Design review of the part built by this model. Coordinates are the model's own, in mm. Face numbers are marked on the shaded views. A direction names the side the tool comes from. Give positions to 0.01 mm unless a question says otherwise; leave off trailing zeros. Loops run counter-clockwise (first coordinate to the right, second up) from the corner with the lowest first, then second, coordinate; pieces in that order, holes last. Notation, with made-up numbers: (19.5, 24.25) -> (62.5, 24.25) arc R24 cw to (62.5, 56.25) -> close; hole circle Ø10 at (6, -9). An arc over 180 degrees is marked (long way). Use a Markdown table: item, result. Add a question column.
1. To check wall thickness, follow line 1 (Y direction, x = 0, z = 11); line 2 (Y direction, x = 0, z = 0.7). State the ranges of each line that lie inside material, in increasing order.
2. For pin 1 Ø3 at (y, z) = (24, 6.5) entering from -X; pin 2 Ø4 at (y, z) = (22.5, 9) entering from +X; pin 3 Ø1 at (x, y) = (8, -16.5) entering from +Z; pin 4 Ø3 at (x, z) = (-22.5, 4) entering from +Y, all flat-tipped, find the tip position at first contact; note any pin that passes through.
3. Add section A-A (x = 0). State the section outline as (y, z) points, and give its area (3 significant figures).
4. Add section C-C (z = 3.5). State the section outline as (x, y) points, and give its area (3 significant figures).
5. Draft analysis for pull direction X (two halves, no side actions). For the marked faces 1, 2, 3 and 4, state which applies: pulls with the +X half, pulls with the -X half, needs draft (parallel to the pull), parting line crosses it, or undercut.
6. For the marked faces 5, 6, 7, 8 and 9, list the 3-axis set-ups (+Z, -Z, +X, -X, +Y, -Y) from which the entire face can be reached by the end or side of a thin tool; tool diameter is ignored.
Autodesk Inventor part; units mm, degrees
ref_plane "YZ Plane" through (0, 0, 0) normal (1, 0, 0) x (0, 1, 0)
ref_plane "XZ Plane" through (0, 0, 0) normal (0, 1, 0) x (-1, 0, 0)
ref_plane "XY Plane" through (0, 0, 0) normal (0, 0, 1) x (1, 0, 0)
sketch "Sketch1" plane through (0, 0, 0) normal (0, 0, 1) x (1, 0, 0)
  line L0 (-34.8609, 0) -> (34.8609, 0) construction
  line L1 (0, -34.8609) -> (0, 34.8609) construction
  line L2 (0, 0) -> (13.4339, 13.4339) construction
  line L3 (0, 0) -> (18.9985, 0) construction
  line L4 (0, 24.9006) -> (16.8, 24.9006)
  line L5 (16.8, 24.9006) -> (16.8, 21.2406)
  line L6 (16.8, 21.2406) -> (19.0203, 19.0203)
  line L7 (24.9006, 0) -> (24.9006, 16.8)
  line L8 (24.9006, 16.8) -> (21.2406, 16.8)
  line L9 (21.2406, 16.8) -> (19.0203, 19.0203)
  line L10 (0, 0) -> (-13.4339, 13.4339) construction
  line L11 (0, 0) -> (-18.9985, 0) construction
  line L12 (0, 24.9006) -> (-16.8, 24.9006)
  line L13 (-16.8, 24.9006) -> (-16.8, 21.2406)
  line L14 (-16.8, 21.2406) -> (-19.0203, 19.0203)
  line L15 (-24.9006, 0) -> (-24.9006, 16.8)
  line L16 (-24.9006, 16.8) -> (-21.2406, 16.8)
  line L17 (-21.2406, 16.8) -> (-19.0203, 19.0203)
  line L18 (0, 0) -> (13.4339, -13.4339) construction
  line L19 (0, -24.9006) -> (16.8, -24.9006)
  line L20 (16.8, -24.9006) -> (16.8, -21.2406)
  line L21 (16.8, -21.2406) -> (19.0203, -19.0203)
  line L22 (24.9006, 0) -> (24.9006, -16.8)
  line L23 (24.9006, -16.8) -> (21.2406, -16.8)
  line L24 (21.2406, -16.8) -> (19.0203, -19.0203)
  line L25 (0, 0) -> (-13.4339, -13.4339) construction
  line L26 (0, -24.9006) -> (-16.8, -24.9006)
  line L27 (-16.8, -24.9006) -> (-16.8, -21.2406)
  line L28 (-16.8, -21.2406) -> (-19.0203, -19.0203)
  line L29 (-24.9006, 0) -> (-24.9006, -16.8)
  line L30 (-24.9006, -16.8) -> (-21.2406, -16.8)
  line L31 (-21.2406, -16.8) -> (-19.0203, -19.0203)
  dimension "d0" = 45
  dimension "d1" = 3.14
  dimension "d2" = 3.66
  dimension "d3" = 16.8
extrude "Thickness" add sketch "Sketch1" along normal blind 14
hole "Hole1" at (0, 0, 0) direction (0, 0, 1) diameter 41.2 end through all
sketch "Sketch2" plane through (0, 0, 0) normal (0, 0, -1) x (-1, 0, 0)
  circle A0 centre (0, 0) radius 20.6
  line L0 (16.8, 24.9006) -> (-16.8, 24.9006)
  line L1 (-16.8, 24.9006) -> (-16.8, 21.2406)
  line L2 (-16.8, 21.2406) -> (-21.2406, 16.8)
  line L3 (-21.2406, 16.8) -> (-24.9006, 16.8)
  line L4 (-24.9006, 16.8) -> (-24.9006, -16.8)
  line L5 (-24.9006, -16.8) -> (-21.2406, -16.8)
  line L6 (-21.2406, -16.8) -> (-16.8, -21.2406)
  line L7 (-16.8, -21.2406) -> (-16.8, -24.9006)
  line L8 (-16.8, -24.9006) -> (16.8, -24.9006)
  line L9 (16.8, -24.9006) -> (16.8, -21.2406)
  line L10 (16.8, -21.2406) -> (21.2406, -16.8)
  line L11 (21.2406, -16.8) -> (24.9006, -16.8)
  line L12 (24.9006, -16.8) -> (24.9006, 16.8)
  line L13 (24.9006, 16.8) -> (21.2406, 16.8)
  line L14 (21.2406, 16.8) -> (16.8, 21.2406)
  line L15 (16.8, 21.2406) -> (16.8, 24.9006)
  circle A1 centre (0, 0) radius 19.6
  dimension "d17" = 1
extrude "Extrusion2" add sketch "Sketch2" against normal blind 1 contours A0
sketch "Sketch3" plane through (0, 0, 0) normal (0, 0, -1) x (-1, 0, 0)
  circle A0 centre (0, 0) radius 20.6
  line L0 (-16.8, 24.9006) -> (16.8, 24.9006)
  line L1 (16.8, 24.9006) -> (16.8, 21.2406)
  line L2 (16.8, 21.2406) -> (21.2406, 16.8)
  line L3 (21.2406, 16.8) -> (24.9006, 16.8)
  line L4 (24.9006, 16.8) -> (24.9006, -16.8)
  line L5 (24.9006, -16.8) -> (21.2406, -16.8)
  line L6 (21.2406, -16.8) -> (16.8, -21.2406)
  line L7 (16.8, -21.2406) -> (16.8, -24.9006)
  line L8 (16.8, -24.9006) -> (-16.8, -24.9006)
  line L9 (-16.8, -24.9006) -> (-16.8, -21.2406)
  line L10 (-16.8, -21.2406) -> (-21.2406, -16.8)
  line L11 (-21.2406, -16.8) -> (-24.9006, -16.8)
  line L12 (-24.9006, -16.8) -> (-24.9006, 16.8)
  line L13 (-24.9006, 16.8) -> (-21.2406, 16.8)
  line L14 (-21.2406, 16.8) -> (-16.8, 21.2406)
  line L15 (-16.8, 21.2406) -> (-16.8, 24.9006)
  line L16 (16.8994, 25) -> (-16.8994, 25)
  line L17 (-16.8994, 25) -> (-16.8994, 21.2818)
  line L18 (-16.8994, 21.2818) -> (-21.2818, 16.8994)
  line L19 (-21.2818, 16.8994) -> (-25, 16.8994)
  line L20 (-25, 16.8994) -> (-25, -16.8994)
  line L21 (-25, -16.8994) -> (-21.2818, -16.8994)
  line L22 (-21.2818, -16.8994) -> (-16.8994, -21.2818)
  line L23 (-16.8994, -21.2818) -> (-16.8994, -25)
  line L24 (-16.8994, -25) -> (16.8994, -25)
  line L25 (16.8994, -25) -> (16.8994, -21.2818)
  line L26 (16.8994, -21.2818) -> (21.2818, -16.8994)
  line L27 (21.2818, -16.8994) -> (25, -16.8994)
  line L28 (25, -16.8994) -> (25, 16.8994)
  line L29 (25, 16.8994) -> (21.2818, 16.8994)
  line L30 (21.2818, 16.8994) -> (16.8994, 21.2818)
  line L31 (16.8994, 21.2818) -> (16.8994, 25)
  dimension "d22" = 50
extrude "Extrusion3" add sketch "Sketch3" against normal up to surface (14 mm away) contours L31 L30 L29 L28 L27 L26 L25 L24 L23 L22 L21 L20 L19 L18 L17 L16
ref_plane "Arbeitsebene1" through (0, -16.8994, 0) normal (-1, 0, 0) x (0, 0, 1)
ref_plane "Arbeitsebene2" through (-16.8994, 0, 0) normal (0, 1, 0) x (1, 0, 0)
equation "\"Lens_diameter\" = 25.4"
properties part number "20_Lens_holder_DIA_50mm"
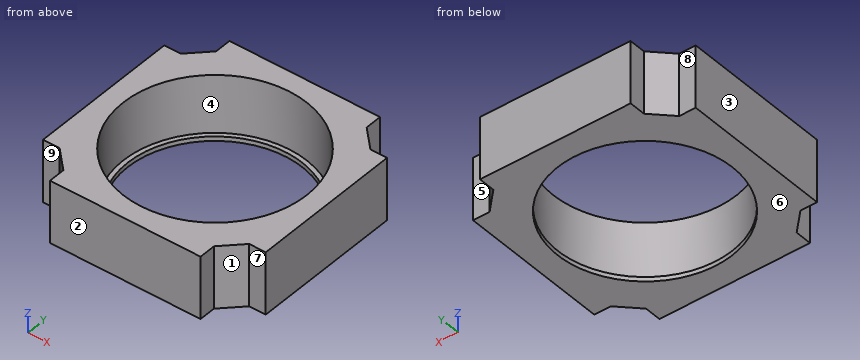
Taken from the geometry:
| question | item | result |
|---|---|---|
| 1 | line 1 | y = -25 to -20.6, 20.6 to 25 |
| 1 | line 2 | y = -25 to -19.6, 19.6 to 25 |
| 2 | pin 1 | stops at x = -16.9 |
| 2 | pin 2 | stops at x = 17.68 |
| 2 | pin 3 | passes through |
| 2 | pin 4 | stops at y = 17.18 |
| 3 | outline | (-25, 0) -> (-19.6, 0) -> (-19.6, 1) -> (-20.6, 1) -> (-20.6, 14) -> (-25, 14) -> close; (19.6, 0) -> (25, 0) -> (25, 14) -> (20.6, 14) -> (20.6, 1) -> (19.6, 1) -> close |
| 3 | area | 125 mm^2 |
| 4 | outline | (-25, -16.9) -> (-21.28, -16.9) -> (-16.9, -21.28) -> (-16.9, -25) -> (16.9, -25) -> (16.9, -21.28) -> (21.28, -16.9) -> (25, -16.9) -> (25, 16.9) -> (21.28, 16.9) -> (16.9, 21.28) -> (16.9, 25) -> (-16.9, 25) -> (-16.9, 21.28) -> (-21.28, 16.9) -> (-25, 16.9) -> close; hole circle Ø41.2 at (0, 0) |
| 4 | area | 943 mm^2 |
| 5 | face 1 | pulls with the +X half |
| 5 | face 2 | needs draft |
| 5 | face 3 | pulls with the -X half |
| 5 | face 4 | undercut |
| 6 | face 5 | +Z, -Z, +X, +Y |
| 6 | face 6 | -Z, +X, -X, +Y, -Y |
| 6 | face 7 | +Z, -Z, +X, -Y |
| 6 | face 8 | +Z, -Z, -X, +Y |
| 6 | face 9 | +Z, -Z, -X, -Y |
